from build123d import *

# Parameters (mm, degrees)
F1_DEPTH  = 30
F2_T      = -6
F4_DEPTH  = 6.001
F6_DEPTH  = 3
F8_DEPTH  = 6.001
F10_DEPTH = 3


with BuildPart() as f1:
    # F0 (on Top) → F1 (new body)
    with BuildSketch(Plane.XY):
        Polygon((0, 30), (0, 0), (30, 30), align=None)
    extrude(amount=F1_DEPTH)

    # F2
    f2_openings = [f1.faces().sort_by_distance(p)[0] for p in [
        (15, 15, 15),
    ]]
    offset(amount=F2_T, openings=f2_openings)

    # F3 (on face) → F4 (cut, through all)
    with BuildSketch(Plane.XZ.offset(-24)):
        with BuildLine():
            ThreePointArc((17.5, 13), (19.5, 15), (17.5, 17))
            Line((17.5, 17), (12.5, 17))
            ThreePointArc((12.5, 17), (10.5, 15), (12.5, 13))
            Line((12.5, 13), (17.5, 13))
        make_face()
    extrude(amount=-F4_DEPTH, mode=Mode.SUBTRACT)

    # F5 (on face) → F6 (cut)
    with BuildSketch(Plane.XZ.offset(-24)):
        with BuildLine():
            ThreePointArc((17.5, 10), (22.5, 15), (17.5, 20))
            Line((17.5, 20), (12.5, 20))
            ThreePointArc((12.5, 20), (7.5, 15), (12.5, 10))
            Line((12.5, 10), (17.5, 10))
        make_face()
    extrude(amount=-F6_DEPTH, mode=Mode.SUBTRACT)

    # F7 (on face) → F8 (cut, through all)
    with BuildSketch(Plane.YZ.offset(6)):
        with BuildLine():
            ThreePointArc((17.5, 13), (19.5, 15), (17.5, 17))
            Line((17.5, 17), (12.5, 17))
            ThreePointArc((12.5, 17), (10.5, 15), (12.5, 13))
            Line((12.5, 13), (17.5, 13))
        make_face()
    extrude(amount=-F8_DEPTH, mode=Mode.SUBTRACT)

    # F9 (on face) → F10 (cut)
    with BuildSketch(Plane.YZ.offset(6)):
        with BuildLine():
            ThreePointArc((12.5, 20), (7.5, 15), (12.5, 10))
            Line((12.5, 10), (17.5, 10))
            ThreePointArc((17.5, 10), (22.5, 15), (17.5, 20))
            Line((17.5, 20), (12.5, 20))
        make_face()
    extrude(amount=-F10_DEPTH, mode=Mode.SUBTRACT)


solid = f1.part
Design review of the part built by this model. Coordinates are the model's own, in mm. A direction names the side the tool comes from. Give positions to 0.01 mm unless a question says otherwise; leave off trailing zeros. Loops run counter-clockwise (first coordinate to the right, second up) from the corner with the lowest first, then second, coordinate; pieces in that order, holes last. Notation, with made-up numbers: M 18.5,-29.75 L 75.5,-29.75 A16 cw 75.5,-1.75 Z; hole C 38.5,-2.5 d1. An arc over 180 degrees is marked long. Write item = value, one per line.
Q1. We need section C-C (x = 6.5). Give the boundary of the cut face in (y, z), plus the area to 3 significant figures.
Output values:
outline = M 6.5,0 L 30,0 L 30,30 L 6.5,30 L 6.5,24 L 24,24 L 24,6 L 6.5,6 Z
area = 390 mm^2
Q2. We need section B-B (y = 28). Give the boundary of the cut face in (x, z).
Output values:
outline = M 0,0 L 28,0 L 28,30 L 0,30 Z; hole M 12.5,13 L 17.5,13 A2 ccw 17.5,17 L 12.5,17 A2 ccw Z
Q3. We need section D-D (y = 23.5). Give the boundary of the cut face in (x, z), plus the area to 3 significant figures.
Output values:
outline = M 0,0 L 23.5,0 L 23.5,6 L 6,6 L 6,24 L 23.5,24 L 23.5,30 L 0,30 Z
area = 390 mm^2
Q4. Insertion check: pin 1 (8 mm diameter, centred on x = 14.5, y = 5, fed in from +Z); pin 2 (9 mm diameter, centred on x = 11, y = 13.5, fed in from -Z); pin 3 (9 mm diameter, centred on y = 13.5, z = 11, fed in from +X); pin 4 (9 mm diameter, centred on x = 12.5, z = 14, fed in from -Y). Each pin has a flat end and moves straight along its axis. Give the tip position at first contact, or say it passes through.
Output values:
pin_1 = through
pin_2 = 0
pin_3 = 6
pin_4 = 24
Q5. For faces 4 (the flat face through (14.9, 27, 12.8)), 5 (the flat face through (13, 17, 6)), 6 (the cylindrical face through (1.5, 19.5, 15)), list the 3-axis set-ups (+Z, -Z, +X, -X, +Y, -Y) from which the entire face can be reached by the end or side of a thin tool; tool diameter is ignored.
Output values:
face_4 = -Y
face_5 = +X, -Y
face_6 = +X, -X
Q6. We need section A-A (z = 15). Give the boundary of the cut face in (x, y), plus the area to 3 significant figures.
Output values:
outline = M 0,0 L 6,6 L 6,7.5 L 3,7.5 L 3,10.5 L 0,10.5 Z; M 0,19.5 L 3,19.5 L 3,22.5 L 6,22.5 L 6,24 L 7.5,24 L 7.5,27 L 10.5,27 L 10.5,30 L 0,30 Z; M 19.5,27 L 22.5,27 L 22.5,24 L 24,24 L 30,30 L 19.5,30 Z
area = 144 mm^2
Q7. To check wall thickness, follow line 1 (Z direction, x = 12.5, y = 25.5); line 2 (Z direction, x = 12.5, y = 18.5); line 3 (X direction, y = 9.5, z = 10.5). State the ranges of each line that lie inside material, in increasing order. Write a range as [from, to].
Output values:
line_1 = [0, 10], [20, 30]
line_2 = [0, 6], [24, 30]
line_3 = [0, 6]
Q8. Draft analysis for pull direction X (two halves, no side actions). For faces 1 (the flat face through (3, 14.9, 12.8)), 2 (the cylindrical face through (1.5, 10.5, 15)), 3 (the flat face through (15, 28, 17)), state which applies: +X half, -X half, draft (parallel to the pull), parting line (faces both ways), or undercut.
Output values:
face_1 = +X half
face_2 = draft
face_3 = undercut
